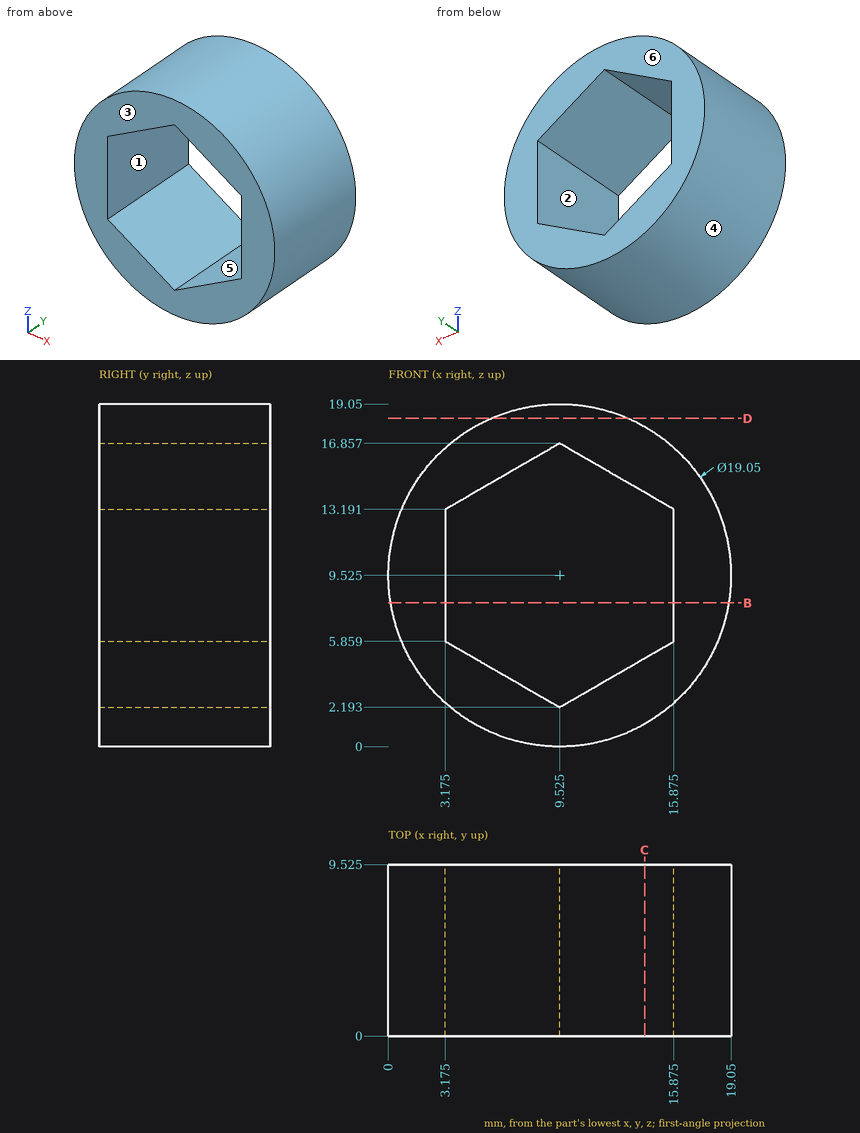
Check sheet for the drawn part. Datum: minimum x, y, z corner. Units: mm. A direction names the side the tool comes from. Coordinates: 2 decimals unless noted, no trailing zeros. Loops run counter-clockwise (first coordinate to the right, second up) from the corner with the lowest first, then second, coordinate; pieces in that order, holes last. Notation, with made-up numbers: (87.5, 57) -> (137.5, 57) arc R24 ccw to (137.5, 82) -> close; hole circle Ø1 at (15, 65.5). An arc over 180 degrees is marked (long way). Answer as a JSON object with one key per item and string values. Group by question number.
Item 1: Mould release check, pull along Z, two halves, no side actions. Record for the marked faces 1, 2, 3 and 4: +Z half, -Z half, draft (parallel to the pull), parting line (faces both ways), or undercut.
Item 2: Sectioned sample at D-D on z = 18.25. Record the boundary of the cut face in (x, y) (1 decimal).
Item 3: Tool access check on the marked faces 5 and 6. Record the directions out of +Z, -Z, +X, -X, +Y, -Y that give a thin tool (end or side, any length) a straight path to the whole face; none if there is none.
Item 4: Scan lines: probe 1 along Z at (x, y) = (11.5, 2.25); probe 2 along X at (y, z) = (2, 9.25) (1 decimal); probe 3 along Z at (x, y) = (9.25, 3.75) (1 decimal). Record each from-to range of solid material in increasing order.
Item 5: Depth check by flat-ended pin: pin 1 (5 mm diameter, centred on x = 8, y = 4.5, fed in from +Z); pin 2 (4 mm diameter, centred on x = 12, y = 2.5, fed in from -Z). Enter the tip coordinate at first touch or a pass-through.
Item 6: Sectioned sample at C-C on x = 14.25. Record the boundary of the cut face in (y, z) (1 decimal).
Item 7: Sectioned sample at B-B on z = 8. Record the boundary of the cut face in (x, y) (1 decimal).
Evaluation:
{
 "1": {"face 1": "undercut", "face 2": "undercut", "face 3": "draft", "face 4": "parting line"},
 "2": {"outline": "(5.7, 0) -> (13.3, 0) -> (13.3, 9.5) -> (5.7, 9.5) -> close"},
 "3": {"face 5": "+Y, -Y", "face 6": "+Z, -Z, +X, -X, +Y"},
 "4": {"probe 1": "z = 0.21 to 3.33, 15.72 to 18.84", "probe 2": "x = 0 to 3.2, 15.9 to 19", "probe 3": "z = 0 to 2.4, 16.7 to 19"},
 "5": {"pin 1": "stops at z = 19.05", "pin 2": "stops at z = 0.01"},
 "6": {"outline": "(0, 1.3) -> (9.5, 1.3) -> (9.5, 4.9) -> (0, 4.9) -> close; (0, 14.1) -> (9.5, 14.1) -> (9.5, 17.8) -> (0, 17.8) -> close"},
 "7": {"outline": "(0.1, 0) -> (3.2, 0) -> (3.2, 9.5) -> (0.1, 9.5) -> close; (15.9, 0) -> (18.9, 0) -> (18.9, 9.5) -> (15.9, 9.5) -> close"}
}
